Autodesk Inventor part; units mm, degrees
ref_plane "YZ Plane" through (0, 0, 0) normal (1, 0, 0) x (0, 1, 0)
ref_plane "XZ Plane" through (0, 0, 0) normal (0, 1, 0) x (-1, 0, 0)
ref_plane "XY Plane" through (0, 0, 0) normal (0, 0, 1) x (1, 0, 0)
sketch "Sketch1" plane through (0, 0, 0) normal (0, 0, 1) x (1, 0, 0)
  line L0 (0, 0) -> (30, 0)
  line L1 (30, 0) -> (30, 4)
  line L2 (30, 4) -> (68, 4)
  line L3 (68, 4) -> (68, 20)
  line L4 (68, 20) -> (24, 20)
  line L5 (24, 20) -> (24, 16)
  line L6 (24, 16) -> (0, 16)
  line L7 (0, 16) -> (0, 0)
  dimension "d0" = 30
  dimension "d1" = 4
  dimension "d2" = 38
  dimension "d3" = 16
  dimension "d4" = 44
  dimension "d5" = 4
extrude "Extrusion1" add sketch "Sketch1" against normal blind 82
sketch "Sketch2" plane through (24, 20, 0) normal (0, 1, 0) x (1, 0, 0)
  circle A0 centre (32, 12) radius 5
  circle A1 centre (32, 70) radius 5
  line L0 (44, 0) -> (44, 82)
  line L1 (44, 0) -> (0, 0)
  line L2 (0, 82) -> (44, 82)
  point P0 (-24, 0)
  dimension "d8" = 10
  dimension "d9" = 10
  dimension "d10" = 12
  dimension "d11" = 12
  dimension "d12" = 12
  dimension "d13" = 12
extrude "Extrusion2" cut sketch "Sketch2" against normal blind 82 contours A0
extrude "Extrusion3" cut sketch "Sketch2" against normal blind 82 contours A1
fillet "Fillet1" radius 12 1 edges at (68, 12, 0)
fillet "Fillet2" radius 12 1 edges at (68, 12, -82)
mirror "Mirror1" about plane through (0, 0, 0) normal (1, 0, 0) of "Extrusion1", "Fillet1", "Extrusion2", "Extrusion3", "Fillet2"
properties part number "topPlate" material "Iron, Malleable"
Input: part model. Units: mm. Frame: model coordinates. A direction names the side the tool comes from. Give positions to 0.01 mm unless a question says otherwise; leave off trailing zeros. Loops run counter-clockwise (first coordinate to the right, second up) from the corner with the lowest first, then second, coordinate; pieces in that order, holes last. Notation, with made-up numbers: (45.5, -8) -> (82.5, -8) arc R35 ccw to (82.5, 25) -> close; hole circle Ø2 at (-21.5, 47.5). An arc over 180 degrees is marked (long way). Use a Markdown table: item, result.
Q1. First-contact query: P1, Ø1.5, axis at x = 9, z = -21, coming from the -Y side; P2, Ø24, axis at x = -8, z = -37, coming from the +Y side; P3, Ø2, axis at x = 39.5, z = -50, coming from the -Y side; P4, Ø8, axis at x = -56, z = -12, coming from the +Y side. Flat tips, straight axial feed; report the tip coordinate or a pass-through.
Entries:
| item | result |
|---|---|
| P1 | stops at y = 0 |
| P2 | stops at y = 16 |
| P3 | stops at y = 4 |
| P4 | passes through |
Q2. Access query for faces 4 (the flat face through (0, 16, -40)), 5 (the flat face through (-30, 2, -40)), 6 (the flat face through (30, 2, -40)). Directions: +Z, -Z, +X, -X, +Y, -Y. A direction counts if a zero-diameter tool reaches every point of the face in a straight line with its end or side. Return the directions, or none.
Entries:
| item | result |
|---|---|
| face 4 | +Z, -Z, +Y |
| face 5 | +Z, -Z, -X, -Y |
| face 6 | +Z, -Z, +X, -Y |
Q3. Section query C-C, the plane y = 8.25. Return the cut outline in (x, z), plus the area to 3 significant figures.
Entries:
| item | result |
|---|---|
| outline | (-68, -70) arc R12 ccw to (-56, -82) -> (56, -82) arc R12 ccw to (68, -70) -> (68, -12) arc R12 ccw to (56, 0) -> (-56, 0) arc R12 ccw to (-68, -12) -> close; hole circle Ø10 at (-56, -70); hole circle Ø10 at (-56, -12); hole circle Ø10 at (56, -70); hole circle Ø10 at (56, -12) |
| area | 10,700 mm² |
Q4. Ray query, probe 1 along Z at (x, y) = (-56, 12.5); probe 2 along X at (y, z) = (14.5, -12); probe 3 along X at (y, z) = (6.25, -14). Return the intervals inside material, ascending. Write a range as from..to.
Entries:
| item | result |
|---|---|
| probe 1 | z = -82..-75, -65..-17, -7..0 |
| probe 2 | x = -68..-61, -51..51, 61..68 |
| probe 3 | x = -68..-60.58, -51.42..51.42, 60.58..68 |
Q5. Section query B-B, the plane z = -19. Return the cut outline in (x, y), plus the area to 3 significant figures.
Entries:
| item | result |
|---|---|
| outline | (-68, 4) -> (-30, 4) -> (-30, 0) -> (30, 0) -> (30, 4) -> (68, 4) -> (68, 20) -> (24, 20) -> (24, 16) -> (-24, 16) -> (-24, 20) -> (-68, 20) -> close |
| area | 2,220 mm² |
Q6. Section query A-A, the plane y = 17.5. Return the cut outline in (x, z), plus the area to 3 significant figures.
Entries:
| item | result |
|---|---|
| outline | (-68, -70) arc R12 ccw to (-56, -82) -> (-24, -82) -> (-24, 0) -> (-56, 0) arc R12 ccw to (-68, -12) -> close; (24, -82) -> (56, -82) arc R12 ccw to (68, -70) -> (68, -12) arc R12 ccw to (56, 0) -> (24, 0) -> close; hole circle Ø10 at (-56, -70); hole circle Ø10 at (-56, -12); hole circle Ø10 at (56, -70); hole circle Ø10 at (56, -12) |
| area | 6,780 mm² |
Q7. Section query D-D, the plane x = -38.5. Return the cut outline in (y, z), plus the area to 3 significant figures.
Entries:
| item | result |
|---|---|
| outline | (4, -82) -> (20, -82) -> (20, 0) -> (4, 0) -> close |
| area | 1,310 mm² |
Q8. Pull-direction query (X, two-part tool) for faces 1 (the flat face through (-49, 4, -40)), 2 (the flat face through (24, 18, -40)), 3 (the cylindrical face through (-64.39, 12.11, -78.58)); classes: pulls with the +X half, pulls with the -X half, needs draft (parallel to the pull), parting line crosses it, or undercut.
Entries:
| item | result |
|---|---|
| face 1 | needs draft |
| face 2 | undercut |
| face 3 | pulls with the -X half |
